Can you work these out from the model? Positions are in its coordinate system, mm. A direction names the side the tool comes from. Give positions to 0.01 mm unless a question says otherwise; leave off trailing zeros. Write each loop counter-clockwise with the first axis right and the second up, starting at its lowest first coordinate (ties: lowest second). Pieces come first, ordered by that corner, then holes. Notation, with made-up numbers: (24.5, 27.25) -> (72.5, 27.25) arc R9 ccw to (72.5, 42.25) -> close; hole circle Ø9 at (72, 62). An arc over 180 degrees is marked (long way). Answer as CSV lines item,"result". Start each with the question number.
1. If we section it at A-A on x = 0: Write out the boundary of the cut face in (y, z), plus the area to 3 significant figures.
2. If we section it at D-D on x = 9: Write out the boundary of the cut face in (y, z).
3. If we section it at B-B on y = 0: Write out the boundary of the cut face in (x, z).
4. If we section it at C-C on z = 11.5: Write out the boundary of the cut face in (x, y), plus the area to 3 significant figures.
5. On a 3-axis mill with a long thin cutter (end or side, diameter ignored), from which of +Z, -Z, +X, -X, +Y, -Y can I reach the whole of each face in a straight line? I mean faces 5 (the face through (14, -7.404, 3)), 6 (the face through (-16, -6, 7)), 7 (the face through (-1.5, 13, 12)), 8 (the face through (2.285, 3.584, 14.726)). Say none if no direction works.
6. I'm going to push flat-ended pins straight in: P1, Ø2, axis at x = -16.5, z = 2, coming from the +Y side; P2, Ø4.5, axis at x = -14.5, z = 2, coming from the -Y side; P3, Ø2, axis at x = 14, z = 3.5, coming from the -Y side; P4, Ø8, axis at x = -13, z = 13, coming from the -Y side. Where does each tip first touch, or does it pass through?
7. If we mould it in two halves opening along X, with no side actions, what happens to faces 1 (the face through (0, 6.696, 7)), 2 (the face through (-14, -15.713, 3)), 3 (the face through (6.5, 6, 6)), 4 (the face through (-12, -7.404, 3))? For each: pulls with the +X half, pulls with the -X half, needs draft (parallel to the pull), parting line crosses it, or undercut.
8. I need wall thicknesses on line 1 (Y direction, x = 0, z = 4.25); line 2 (X direction, y = 14.5, z = 6.5); line 3 (Z direction, x = 0, y = 15). Which ranges of each line are inside material? Lowest first, please. Write a range as [from, to].
```python
from build123d import *

# Parameters (mm, degrees)
F0_W     = 13
F0_H     = 24
F0_H_2   = 3
F2_DEPTH = 13
F1_R     = 2.2
F3_DEPTH = 13
F5_DEPTH = 12.9
F6_DEPTH = 7
F1_R_2   = 4.25
F7_DEPTH = 16.5


with BuildPart() as f2:
    # F0 (on Top) → F2 (new body)
    with BuildSketch(Plane.XY):
        with Locations((0, 7.5963802942)):
            Rectangle(F0_W, F0_H)
        with Locations((0, -5.9036197058)):
            Rectangle(F0_W, F0_H_2)
        with BuildLine():
            Line((6.5, -7.4036197058), (-6.5, -7.4036197058))
            ThreePointArc((-6.5, -7.4036197058), (0, -9.8520852995), (6.5, -7.4036197058))
        make_face()
    extrude(amount=F2_DEPTH)

    # F1 (on Top) → F3 (cut, through all)
    with BuildSketch(Plane.XY):
        Circle(F1_R)
    extrude(amount=F3_DEPTH, mode=Mode.SUBTRACT)

    # F4 (on face) → F5 (cut)
    with BuildSketch(Plane(origin=(0, 19.5963802942, 0), x_dir=(-1, 0, 0), z_dir=(0, 1, 0))):
        with BuildLine():
            ThreePointArc((-1.5, 10.4764934301), (-2.4173849507, 3.0044671365), (4.25, 6.5))
            ThreePointArc((4.25, 6.5), (3.4955328635, 8.9173849507), (1.5, 10.4764934301))
            ThreePointArc((1.5, 10.4764934301), (0, 10.75), (-1.5, 10.4764934301))
        make_face()
        with BuildLine():
            ThreePointArc((-1.5, 10.4764934301), (0, 10.75), (1.5, 10.4764934301))
            Line((1.5, 10.4764934301), (1.5, 13))
            Line((1.5, 13), (-1.5, 13))
            Line((-1.5, 13), (-1.5, 10.4764934301))
        make_face()
    extrude(amount=-F5_DEPTH, mode=Mode.SUBTRACT)

    # F0 (on Top) → F6 (join)
    with BuildSketch(Plane.XY):
        with BuildLine():
            Line((24.700689028, -4.4036197058), (6.5, -4.4036197058))
            Line((6.5, -4.4036197058), (6.5, -7.4036197058))
            Line((6.5, -7.4036197058), (20.9526508047, -7.4036197058))
            ThreePointArc((20.9526508047, -7.4036197058), (18.798000482, -11.8516808248), (15.7134840264, -15.7134840264))
            Line((15.7134840264, -15.7134840264), (16.2143083706, -19.1471175125))
            ThreePointArc((16.2143083706, -19.1471175125), (21.7451588848, -12.5165478486), (24.700689028, -4.4036197058))
        make_face()
        with BuildLine():
            Line((-6.5, -7.4036197058), (-6.5, -4.4036197058))
            Line((-6.5, -4.4036197058), (-21.7815356203, -4.4036197058))
            ThreePointArc((-21.7815356203, -4.4036197058), (-19.581812539, -10.5061780958), (-15.7134840264, -15.7134840264))
            Line((-15.7134840264, -15.7134840264), (-11.7134840264, -15.7134840264))
            ThreePointArc((-11.7134840264, -15.7134840264), (-15.4974944993, -11.9977894851), (-18.1467821813, -7.4036197058))
            Line((-18.1467821813, -7.4036197058), (-6.5, -7.4036197058))
        make_face()
    extrude(amount=F6_DEPTH)

    # F1 (on Top) → F7 (join)
    with BuildSketch(Plane.XY):
        Circle(F1_R_2)
        Circle(F1_R, mode=Mode.SUBTRACT)
    extrude(amount=F7_DEPTH)


solid = f2.part
```
Computed values:
1,outline,"(-9.85, 0) -> (-2.2, 0) -> (-2.2, 16.5) -> (-4.25, 16.5) -> (-4.25, 13) -> (-9.85, 13) -> close; (2.2, 0) -> (19.6, 0) -> (19.6, 2.25) -> (6.7, 2.25) -> (6.7, 13) -> (4.25, 13) -> (4.25, 16.5) -> (2.2, 16.5) -> close"
1,area,"201 mm2"
2,outline,"(-7.4, 0) -> (-4.4, 0) -> (-4.4, 7) -> (-7.4, 7) -> close"
3,outline,"(-6.5, 0) -> (-2.2, 0) -> (-2.2, 16.5) -> (-4.25, 16.5) -> (-4.25, 13) -> (-6.5, 13) -> close; (2.2, 0) -> (6.5, 0) -> (6.5, 13) -> (4.25, 13) -> (4.25, 16.5) -> (2.2, 16.5) -> close"
4,outline,"(-6.5, -7.4) arc R9.85 ccw to (6.5, -7.4) -> (6.5, 19.6) -> (1.5, 19.6) -> (1.5, 6.7) -> (-1.5, 6.7) -> (-1.5, 19.6) -> (-6.5, 19.6) -> close; hole circle Ø4.4 at (0, 0)"
4,area,"319 mm2"
5,face 5,"+Z, -Z"
5,face 6,"+Z, -X, +Y, -Y"
5,face 7,"+Z, +Y"
5,face 8,"+Z"
6,P1,"stops at y = -4.4"
6,P2,"stops at y = -15.71"
6,P3,"stops at y = -7.4"
6,P4,"passes through"
7,face 1,"undercut"
7,face 2,"needs draft"
7,face 3,"pulls with the +X half"
7,face 4,"undercut"
8,line 1,"y = [-9.85, -2.2], [2.2, 6.7]"
8,line 2,"x = [-6.5, -4.25], [4.25, 6.5]"
8,line 3,"z = [0, 2.25]"
